Geometry check sheet. Reference: the model listing, model coordinates, mm. Give positions to 0.01 mm unless a question says otherwise; leave off trailing zeros. Loops run counter-clockwise (first coordinate to the right, second up) from the corner with the lowest first, then second, coordinate; pieces in that order, holes last. Notation, with made-up numbers: (13, 63.25) -> (25, 63.25) arc R4 cw to (25, 68.25) -> close; hole circle Ø3 at (-21, 70.5). An arc over 180 degrees is marked (long way). Write item = value, one per line.
```python
from build123d import *

# Parameters (mm, degrees)
SKETCH1_R           = 27
SKETCH1_R_2         = 8
SKETCH1_R_3         = 1.75
BOSS_EXTRUDE1_DEPTH = 2
SKETCH2_W           = 15
SKETCH2_H           = 3
CUT_EXTRUDE1_DEPTH  = 39.236108589
FILLET1_R           = 1


with BuildPart() as part:
    # Sketch1 → Boss-Extrude1 (new body)
    with BuildSketch(Plane(origin=(0, 0, 0), x_dir=(1, 0, 0), z_dir=(0, 1, 0))):
        with Locations(Location((0, 0, 0), (0, 0, 270))):
            Circle(SKETCH1_R)
        with Locations(Location((0, 0, 0), (0, 0, 270))):
            Circle(SKETCH1_R_2, mode=Mode.SUBTRACT)
        with Locations(Location((-23, 0, 0), (0, 0, 270))):
            Circle(SKETCH1_R_3, mode=Mode.SUBTRACT)
        with Locations(Location((23, 0, 0), (0, 0, 270))):
            Circle(SKETCH1_R_3, mode=Mode.SUBTRACT)
    extrude(amount=BOSS_EXTRUDE1_DEPTH)

    # Sketch2 → Cut-Extrude1 (cut, through all)
    with BuildSketch(Plane(origin=(0, 2, 0), x_dir=(1, 0, 0), z_dir=(0, 1, 0))):
        with Locations((-12.5, 0)):
            Rectangle(SKETCH2_W, SKETCH2_H)
    extrude(amount=-CUT_EXTRUDE1_DEPTH, mode=Mode.SUBTRACT)

    # Fillet1
    fillet1_edges = [part.edges().sort_by_distance(p)[0] for p in [
        (-7.858116823, 1, 1.5),
        (-7.858116823, 1, -1.5),
        (-20, 1, 1.5),
        (-20, 1, -1.5),
    ]]
    fillet(fillet1_edges, radius=FILLET1_R)


solid = part.part
```
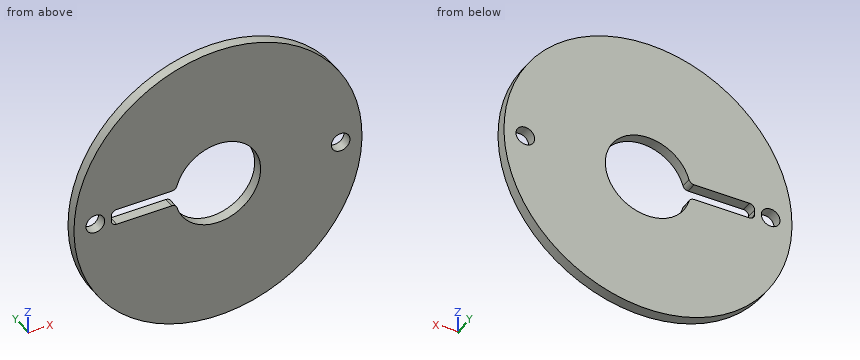
Item 1: Gauge pin test, flat ends, axial feed: pin 1 (1 mm diameter, centred on x = -18.5, y = 1, fed in from +Z); pin 2 (0.6 mm diameter, centred on x = -15.5, y = 0.5, fed in from -Z) (3 decimals); pin 3 (1 mm diameter, centred on y = 1, z = -17.5, fed in from +X). Record the tip position at first contact, or that the pin passes through.
Answer:
pin_1 = 20.12
pin_2 = -22.315
pin_3 = 20.98
Item 2: Section check D-D, the plane z = -13.5. Record the cut outline in (x, y).
Answer:
outline = (-23.38, 0) -> (23.38, 0) -> (23.38, 2) -> (-23.38, 2) -> close
Item 3: Section check C-C, the plane z = -5. Record the cut outline in (x, y) (3 decimals).
Answer:
outline = (-26.533, 0) -> (-6.245, 0) -> (-6.245, 2) -> (-26.533, 2) -> close; (6.245, 0) -> (26.533, 0) -> (26.533, 2) -> (6.245, 2) -> close
Item 4: Thickness scan on L1, parallel to X at y = 0.8, z = 0; L2, parallel to Z at x = 1.5, y = 1.4; L3, parallel to Z at x = -2.5, y = 1.35. Record the ranges inside material, lowest first. Write a range as [from, to].
Answer:
L1 = [-27, -24.75], [-21.25, -20], [8, 21.25], [24.75, 27]
L2 = [-26.96, -7.86], [7.86, 26.96]
L3 = [-26.88, -7.6], [7.6, 26.88]
Item 5: Section check B-B, the plane y = 1.2. Record the cut outline in (x, z).
Answer:
outline = circle Ø54 at (0, 0); hole circle Ø3.5 at (-23, 0); hole (-20, -0.5) arc R1 ccw to (-19, -1.5) -> (-8.65, -1.5) arc R1 cw to (-7.69, -2.22) arc R8 ccw (long way) to (-7.69, 2.22) arc R1 cw to (-8.65, 1.5) -> (-19, 1.5) arc R1 ccw to (-20, 0.5) -> close; hole circle Ø3.5 at (23, 0)
Item 6: Section check A-A, the plane x = 0. Record the cut outline in (y, z).
Answer:
outline = (0, -27) -> (2, -27) -> (2, -8) -> (0, -8) -> close; (0, 8) -> (2, 8) -> (2, 27) -> (0, 27) -> close
